Can you work these out from the model? Positions are in its coordinate system, mm. Face numbers are marked on the shaded views. A direction names the side the tool comes from. Coordinates: 2 decimals unless noted, no trailing zeros. Order: outer loops, then holes, each group sorted by start corner. A loop starts at its lowest first (then second) coordinate and runs counter-clockwise, first axis right, second up. Notation, with made-up numbers: (17.25, 24.5) -> (59.25, 24.5) arc R14 ccw to (59.25, 51.5) -> close; hole circle Ø5 at (71, -17.5). An arc over 180 degrees is marked (long way). Answer in a Markdown table with one row per item. Add a question column.
1. Imagine slicing it at B-B on x = 39. Write out the boundary of the cut face in (y, z), plus the area to 3 significant figures.
2. Imagine slicing it at A-A on y = 125. Write out the boundary of the cut face in (x, z).
3. Will these pins go through, and if not, where does the flat tip stop? pin 1 (1.5 mm diameter, centred on x = 13, y = 32.5, fed in from +Z); pin 2 (10 mm diameter, centred on y = 112, z = -3.5, fed in from +X); pin 3 (5 mm diameter, centred on x = 22, z = 1, fed in from +Y); pin 4 (11.5 mm diameter, centred on x = 0, y = 125, fed in from +Z).
4. We'd pull the mould along X, two halves only. Please class the marked faces 1, 2 and 3: pulls with the +X half, pulls with the -X half, needs draft (parallel to the pull), parting line crosses it, or undercut.
5. On a 3-axis mill with a long thin cutter (end or side, diameter ignored), from which of +Z, -Z, +X, -X, +Y, -Y can I reach the whole of each face in a straight line? I mean the marked faces 4, 5 and 6. Say none if no direction works.
6. If I drill on line 1 along Z through (x, y) = (30, 13); line 2 along Y through (x, z) = (3, -7); line 3 along X through (y, z) = (125, -8.5), over which ranges is the centre line in solid material (lowest first)? Write a range as [from, to].
from build123d import *

# Parameters (mm, degrees)
SKETCH1_R                   = 6.5
BOSS_EXTRUDE1_DEPTH         = 10
SKETCH2_R                   = 14
CUT_EXTRUDE1_DEPTH          = 14
CHAMFER1_SIZE               = 1
CHAMFER1_SIZE2              = 1.732050808
CHAMFER2_SIZE               = 4
CHAMFER2_SIZE2              = 6.92820323
CHAMFER2_PART_2_SIZE        = 4
CHAMFER2_PART_2_SIZE2       = 6.92820323
FILLET1_R                   = 5
CUT_EXTRUDE2_DEPTH          = 4
FILLET2_R                   = 2
FILLET2_OF_MIRROR1_R        = 2
M10X1_25_TAPPED_HOLE1_D     = 8.8
M10X1_25_TAPPED_HOLE1_DEPTH = 20
M10X1_25_TAPPED_HOLE1_TIP   = 2.643786724


with BuildPart() as part:
    # Sketch1 → Boss-Extrude1 (new body, symmetric)
    with BuildSketch(Plane.XY):
        with BuildLine():
            Line((-46, 0), (46, 0))
            Line((46, 0), (46, 15))
            Line((46, 15), (31.449256053, 74.112397284))
            ThreePointArc((31.449256053, 74.112397284), (30.363636327, 80.044097084), (30, 86.06334964))
            Line((30, 86.06334964), (30, 137))
            Line((30, 137), (16, 137))
            ThreePointArc((16, 137), (0, 145), (-16, 137))
            Line((-16, 137), (-30, 137))
            Line((-30, 137), (-30, 86.06334964))
            ThreePointArc((-30, 86.06334964), (-30.363636327, 80.044097084), (-31.449256053, 74.112397284))
            Line((-31.449256053, 74.112397284), (-46, 15))
            Line((-46, 15), (-46, 0))
        make_face()
        with Locations((0, 125)):
            Circle(SKETCH1_R, mode=Mode.SUBTRACT)
    extrude(amount=BOSS_EXTRUDE1_DEPTH, both=True)

    # Sketch2 → Cut-Extrude1 (cut)
    with BuildSketch(Plane.XY.offset(10)):
        with Locations((0, 125)):
            Circle(SKETCH2_R)
    extrude(amount=-CUT_EXTRUDE1_DEPTH, mode=Mode.SUBTRACT)

    # Chamfer1
    chamfer1_edges = [part.edges().sort_by_distance(p)[0] for p in [
        (-14, 125, 10),
    ]]
    chamfer1_side = [part.faces().sort_by_distance(p)[0] for p in [
        (0, 59.441099991, 10),
    ]]
    chamfer(chamfer1_edges, length=CHAMFER1_SIZE, length2=CHAMFER1_SIZE2, reference=chamfer1_side[0])

    # Chamfer2
    chamfer2_edges = [part.edges().sort_by_distance(p)[0] for p in [
        (-30, 137, 0),
    ]]
    chamfer2_side = [part.faces().sort_by_distance(p)[0] for p in [
        (-23, 137, 0),
    ]]
    chamfer(chamfer2_edges, length=CHAMFER2_SIZE, length2=CHAMFER2_SIZE2, reference=chamfer2_side[0])

    # Chamfer2 part 2
    chamfer2_part_2_edges = [part.edges().sort_by_distance(p)[0] for p in [
        (30, 137, 0),
    ]]
    chamfer2_part_2_side = [part.faces().sort_by_distance(p)[0] for p in [
        (30, 111.53167482, 0),
    ]]
    chamfer(chamfer2_part_2_edges, length=CHAMFER2_PART_2_SIZE, length2=CHAMFER2_PART_2_SIZE2, reference=chamfer2_part_2_side[0])

    # Fillet1
    fillet1_edges = [part.edges().sort_by_distance(p)[0] for p in [
        (-16, 137, 0),
        (16, 137, 0),
    ]]
    fillet(fillet1_edges, radius=FILLET1_R)

    # Sketch3 → Cut-Extrude2 (cut)
    with BuildSketch(Plane.XY.offset(10)):
        with BuildLine():
            Line((-18, 92), (-18, 86.06334964))
            ThreePointArc((-18, 86.06334964), (-18.450909046, 78.59947647), (-19.797077506, 71.244168718))
            Line((-19.797077506, 71.244168718), (-29.971112298, 29.912152377))
            ThreePointArc((-29.971112298, 29.912152377), (-28.49970745, 23.065287193), (-22.202993266, 20))
            Line((-22.202993266, 20), (22.202993266, 20))
            ThreePointArc((22.202993266, 20), (28.49970745, 23.065287193), (29.971112298, 29.912152377))
            Line((29.971112298, 29.912152377), (19.797077506, 71.244168718))
            ThreePointArc((19.797077506, 71.244168718), (18.450909046, 78.59947647), (18, 86.06334964))
            Line((18, 86.06334964), (18, 92))
            ThreePointArc((18, 92), (15.656854249, 97.656854249), (10, 100))
            Line((10, 100), (-10, 100))
            ThreePointArc((-10, 100), (-15.656854249, 97.656854249), (-18, 92))
        make_face()
    cut_extrude2 = extrude(amount=-CUT_EXTRUDE2_DEPTH, mode=Mode.SUBTRACT)

    # Fillet2
    fillet2_edges = [part.edges().sort_by_distance(p)[0] for p in [
        (28.49970745, 23.065287193, 6),
        (0, 20, 6),
        (-28.49970745, 23.065287193, 6),
        (-24.884094902, 50.578160548, 6),
        (-18.450909046, 78.59947647, 6),
        (-18, 89.03167482, 6),
        (-15.656854249, 97.656854249, 6),
        (0, 100, 6),
        (15.656854249, 97.656854249, 6),
        (18, 89.03167482, 6),
        (18.450909046, 78.59947647, 6),
        (24.884094902, 50.578160548, 6),
    ]]
    fillet(fillet2_edges, radius=FILLET2_R)

    # Mirror1: Cut-Extrude2 across plane
    add(cut_extrude2.mirror(Plane.XY), mode=Mode.SUBTRACT)

    # Fillet2 of Mirror1
    fillet2_of_mirror1_edges = [part.edges().sort_by_distance(p)[0] for p in [
        (28.49970745, 23.065287193, -6),
        (0, 20, -6),
        (-28.49970745, 23.065287193, -6),
        (-24.884094902, 50.578160548, -6),
        (-18.450909046, 78.59947647, -6),
        (-18, 89.03167482, -6),
        (-15.656854249, 97.656854249, -6),
        (0, 100, -6),
        (15.656854249, 97.656854249, -6),
        (18, 89.03167482, -6),
        (18.450909046, 78.59947647, -6),
        (24.884094902, 50.578160548, -6),
    ]]
    fillet(fillet2_of_mirror1_edges, radius=FILLET2_OF_MIRROR1_R)

    # M10x1.25 Tapped Hole1
    with Locations(Plane(origin=(0, 0, 0), x_dir=(-1, 0, 0), z_dir=(0, -1, 0))):
        with Locations((30, 0), (-30, 0)):
            Hole(M10X1_25_TAPPED_HOLE1_D / 2, depth=M10X1_25_TAPPED_HOLE1_DEPTH)
            with Locations((0, 0, -(M10X1_25_TAPPED_HOLE1_DEPTH + M10X1_25_TAPPED_HOLE1_TIP / 2))):  # 118° drill point
                Cone(0, M10X1_25_TAPPED_HOLE1_D / 2, M10X1_25_TAPPED_HOLE1_TIP, mode=Mode.SUBTRACT)


solid = part.part
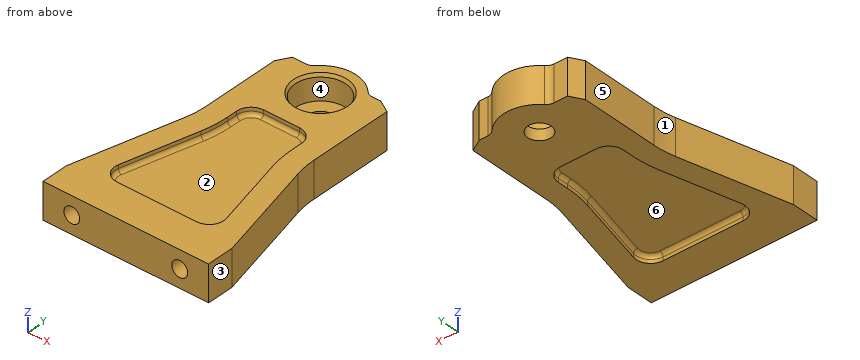
Answers follow:
| question | item | result |
|---|---|---|
| 1 | outline | (0, -10) -> (43.44, -10) -> (43.44, 10) -> (0, 10) -> close |
| 1 | area | 869 mm² |
| 2 | outline | (-30, -10) -> (-6.5, -10) -> (-6.5, -4) -> (-14, -4) -> (-14, 8.27) -> (-15, 10) -> (-30, 10) -> close; (6.5, -10) -> (30, -10) -> (30, 10) -> (15, 10) -> (14, 8.27) -> (14, -4) -> (6.5, -4) -> close |
| 3 | pin 1 | stops at z = 6 |
| 3 | pin 2 | stops at x = 30 |
| 3 | pin 3 | stops at y = 137 |
| 3 | pin 4 | passes through |
| 4 | face 1 | pulls with the -X half |
| 4 | face 2 | undercut |
| 4 | face 3 | pulls with the +X half |
| 5 | face 4 | +Z |
| 5 | face 5 | +Z, -Z, -X, +Y |
| 5 | face 6 | -Z |
| 6 | line 1 | z = [-10, -4.4], [4.4, 10] |
| 6 | line 2 | y = [0, 20.27], [99.73, 119.23], [130.77, 144.77] |
| 6 | line 3 | x = [-30, -6.5], [6.5, 30] |
